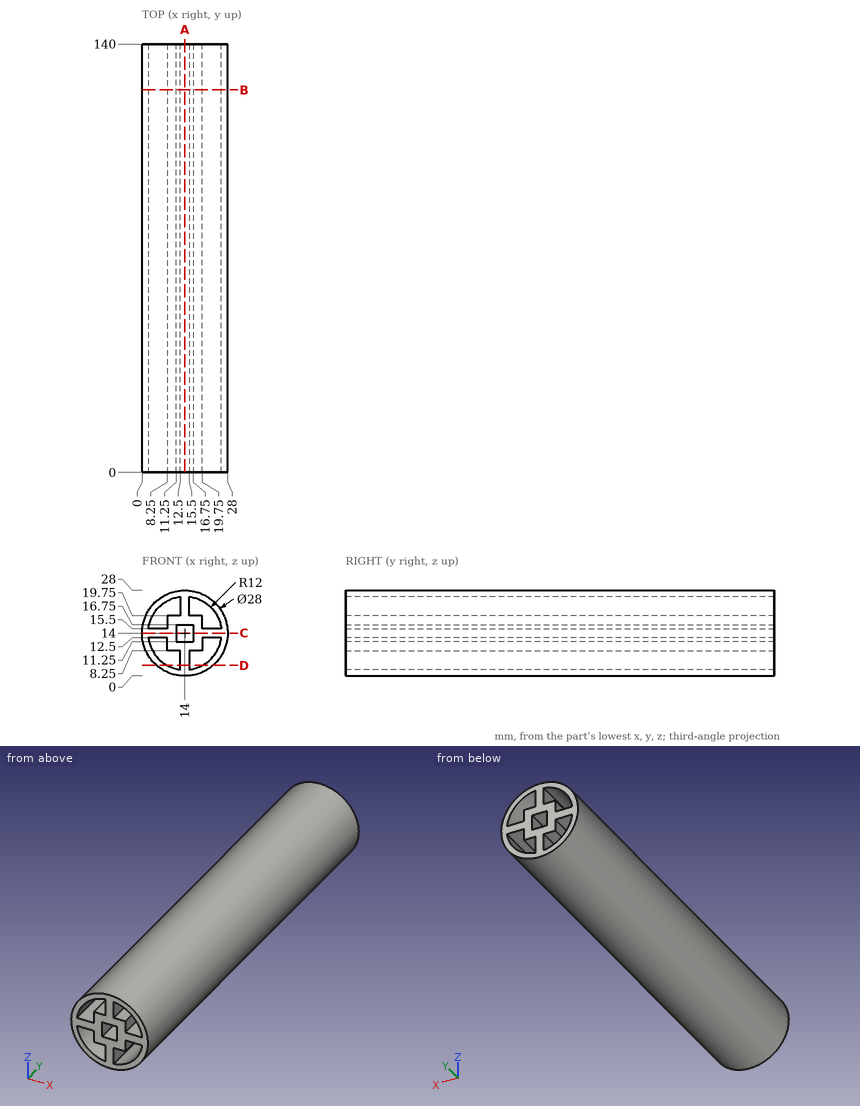
Check sheet for the drawn part. Datum: minimum x, y, z corner. Units: mm. Coordinates: 2 decimals unless noted, no trailing zeros. Loops run counter-clockwise (first coordinate to the right, second up) from the corner with the lowest first, then second, coordinate; pieces in that order, holes last. Notation, with made-up numbers: (75, -14) - (80, -14) arc R31 ccw to (80, 21) - close; hole circle Ø10 at (81.5, 13.5). An arc over 180 degrees is marked (long way). Put each result on its own line as item: value.
Item 1: Section check B-B (y = 125). Enter the section's corners in (x, z).
Conclusion:
outline: circle Ø28 at (14, 14); hole (2.09, 12.5) arc R12 ccw to (12.5, 2.09) - (12.5, 8.25) - (8.25, 8.25) - (8.25, 12.5) - close; hole (2.09, 15.5) - (8.25, 15.5) - (8.25, 19.75) - (12.5, 19.75) - (12.5, 25.91) arc R12 ccw to start; hole (11.25, 11.25) - (16.75, 11.25) - (16.75, 16.75) - (11.25, 16.75) - close; hole (15.5, 2.09) arc R12 ccw to (25.91, 12.5) - (19.75, 12.5) - (19.75, 8.25) - (15.5, 8.25) - close; hole (15.5, 19.75) - (19.75, 19.75) - (19.75, 15.5) - (25.91, 15.5) arc R12 ccw to (15.5, 25.91) - close
Item 2: Gauge pin test, flat ends, axial feed: pin 1 Ø10 at (y, z) = (21, 4.5) entering from +X; pin 2 Ø4 at (x, y) = (24.5, 26) entering from -Z; pin 3 Ø5 at (x, y) = (24, 70) entering from +Z. Record the tip position at first contact, or that the pin passes through.
Conclusion:
pin 1: stops at x = 27.26
pin 2: stops at z = 2.88
pin 3: stops at z = 25.82
Item 3: Section check C-C (z = 14). Enter the section's corners in (x, y), then the cut area to 3 significant figures.
Conclusion:
outline: (0, 0) - (11.25, 0) - (11.25, 140) - (0, 140) - close; (16.75, 0) - (28, 0) - (28, 140) - (16.75, 140) - close
area: 3,150 mm2
Item 4: Scan lines: line 1 along X through (y, z) = (90.5, 13.25); line 2 along X through (y, z) = (118, 11.75); line 3 along X through (y, z) = (10, 5.75). Record each from-to range of solid material in increasing order.
Conclusion:
line 1: x = 0.02 to 11.25, 16.75 to 27.98
line 2: x = 0.18 to 2.21, 8.25 to 11.25, 16.75 to 19.75, 25.79 to 27.82
line 3: x = 2.69 to 5.29, 12.5 to 15.5, 22.71 to 25.31
Item 5: Section check A-A (x = 14). Enter the section's corners in (y, z), then the cut area to 3 significant figures.
Conclusion:
outline: (0, 0) - (140, 0) - (140, 11.25) - (0, 11.25) - close; (0, 16.75) - (140, 16.75) - (140, 28) - (0, 28) - close
area: 3,150 mm2
Item 6: Section check D-D (z = 3.5). Enter the section's corners in (x, y), then the cut area to 3 significant figures.
Conclusion:
outline: (4.74, 0) - (8.19, 0) - (8.19, 140) - (4.74, 140) - close; (12.5, 0) - (15.5, 0) - (15.5, 140) - (12.5, 140) - close; (19.81, 0) - (23.26, 0) - (23.26, 140) - (19.81, 140) - close
area: 1,390 mm2
